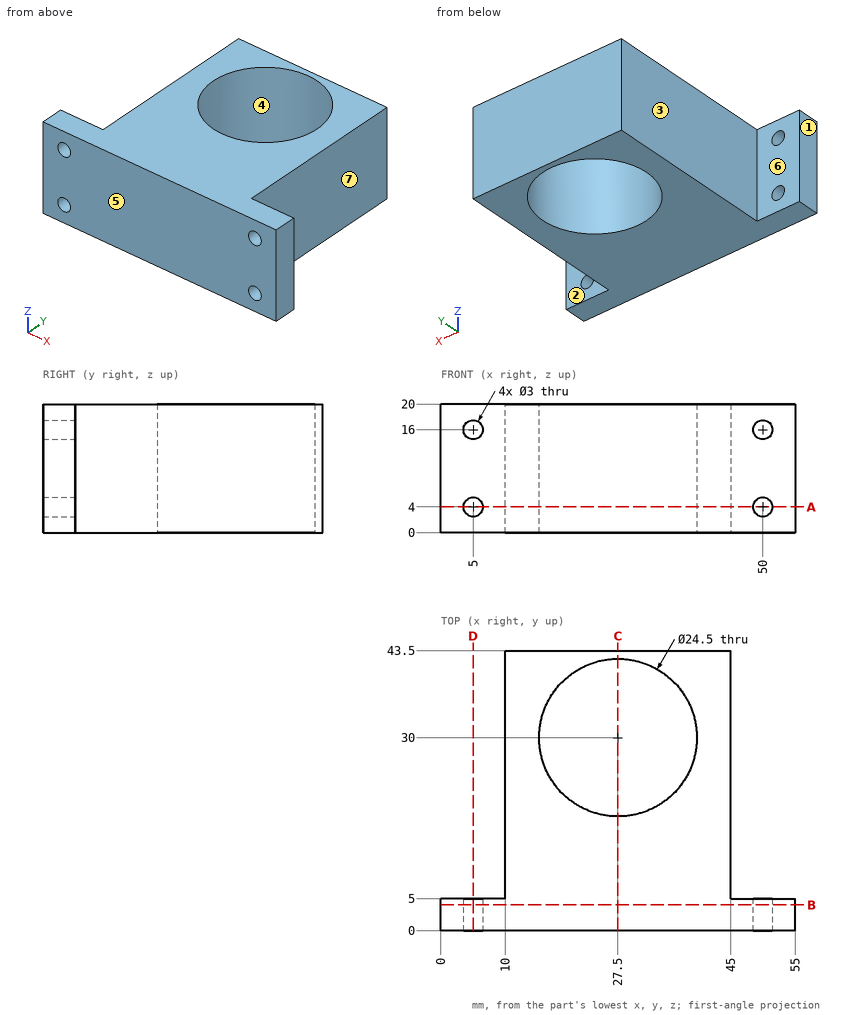
Input: dimensioned drawing with shaded views. Units: mm. Origin: part minimum x, y, z. A direction names the side the tool comes from. Coordinates: 2 decimals unless noted, no trailing zeros. Write each loop counter-clockwise with the first axis right and the second up, starting at its lowest first coordinate (ties: lowest second). Pieces come first, ordered by that corner, then holes. Notation, with made-up numbers: M 57,-1 L 87,-1 A22 ccw 87,27 Z; hole C 72.25,-20 d9. An arc over 180 degrees is marked long. Use one line per item in the form item = value.
Q1. First-contact query: pin 1 (10 mm diameter, centred on y = 23, z = 6, fed in from -X); pin 2 (10 mm diameter, centred on y = 32.5, z = 10.5, fed in from +X); pin 3 (8 mm diameter, centred on x = 21.5, z = 17, fed in from -Y); pin 4 (3 mm diameter, centred on x = 6, z = 8, fed in from +Y). Flat tips, straight axial feed; report the tip coordinate or a pass-through.
Answer below:
pin_1 = 10
pin_2 = 45
pin_3 = 0
pin_4 = 5
Q2. Set-up query: the marked faces 1, 2 and 3. Return all of +Z, -Z, +X, -X, +Y, -Y with unobstructed straight access to the full face (end or side cutting, diameter ignored); none if empty.
Answer below:
face_1 = +Z, -Z, -X, +Y, -Y
face_2 = +Z, -Z, +X, +Y
face_3 = +Z, -Z, -X, +Y
Q3. Draft query along Y for the marked faces 4, 5, 6 and 7. Return one class per face: released by +Y, released by -Y, zero draft, split by the parting line, or undercut.
Answer below:
face_4 = undercut
face_5 = released by -Y
face_6 = released by +Y
face_7 = zero draft
Q4. Section D-D (x = 5). Return loops of the section in (y, z), plus the area to 3 significant figures.
Answer below:
outline = M 0,0 L 5,0 L 5,2.5 L 0,2.5 Z; M 0,5.5 L 5,5.5 L 5,14.5 L 0,14.5 Z; M 0,17.5 L 5,17.5 L 5,20 L 0,20 Z
area = 70.0 mm²
Q5. Section A-A (z = 4). Return loops of the section in (x, y).
Answer below:
outline = M 0,0 L 3.5,0 L 3.5,5 L 0,5 Z; M 6.5,0 L 48.5,0 L 48.5,5 L 45,5 L 45,43.5 L 10,43.5 L 10,5 L 6.5,5 Z; M 51.5,0 L 55,0 L 55,5 L 51.5,5 Z; hole C 27.5,30 d24.5
Q6. Material intervals for probe 1 along Z at (x, y) = (50, 3); probe 2 along X at (y, z) = (2.4, 4); probe 3 along Y at (x, z) = (27.5, 15), sorted ascending. Write a range as from..to.
Answer below:
probe_1 = 0..2.5, 5.5..14.5, 17.5..20
probe_2 = 0..3.5, 6.5..48.5, 51.5..55
probe_3 = 0..17.75, 42.25..43.5
Q7. Section B-B (y = 4). Return loops of the section in (x, z).
Answer below:
outline = M 0,0 L 55,0 L 55,20 L 0,20 Z; hole C 5,4 d3; hole C 5,16 d3; hole C 50,4 d3; hole C 50,16 d3
Q8. Section C-C (x = 27.5). Return loops of the section in (y, z), plus the area to 3 significant figures.
Answer below:
outline = M 0,0 L 17.75,0 L 17.75,20 L 0,20 Z; M 42.25,0 L 43.5,0 L 43.5,20 L 42.25,20 Z
area = 380 mm²
